Autodesk Inventor part; units mm, degrees
ref_plane "YZ Plane" through (0, 0, 0) normal (1, 0, 0) x (0, 1, 0)
ref_plane "XZ Plane" through (0, 0, 0) normal (0, 1, 0) x (-1, 0, 0)
ref_plane "XY Plane" through (0, 0, 0) normal (0, 0, 1) x (1, 0, 0)
ref_plane "РабПлоскость1" through (0, 0, 0) normal (0, 0, 1) x (1, 0, 0)
sketch "Эскиз1" plane through (0, 0, 0) normal (0, 0, 1) x (1, 0, 0)
  circle A0 centre (0, 0) radius 10
  dimension "d0" = 20
extrude "Выдавливание1" add sketch "Эскиз1" against normal blind 90
sketch "Эскиз2" plane through (0, 0, 0) normal (0, 0, 1) x (1, 0, 0)
  circle A0 centre (0, 0) radius 15
  dimension "d3" = 30
extrude "Выдавливание2" add sketch "Эскиз2" along normal blind 30
chamfer "Фаска1" distance 2 angle 45 2 edges at (-15, 0, 30) (-10, 0, -90)
ref_plane "РабПлоскость2" through (-11.5, 3, -60) normal (1, 0, 0) x (0, 1, 0)
sketch "Эскиз3" plane through (-11.5, 3, -60) normal (1, 0, 0) x (0, 1, 0)
  line L0 (-18, 60) -> (12, 60)
  line L1 (12, 88) -> (-18, 88)
  line L2 (-13, 60) -> (7, 60)
  line L3 (-13, -28) -> (7, -28)
  line L4 (-3, 10) -> (-3, 10)
  line L5 (0, 13) -> (0, 47)
  line L6 (-3, 50) -> (-3, 50)
  line L7 (-6, 47) -> (-6, 13)
  line L8 (-6, 10) -> (0, 50) construction
  line L9 (0, 10) -> (-6, 50) construction
  arc A0 (0, 47) -> (-3, 50) centre (-3, 47) ccw
  arc A1 (-3, 50) -> (-6, 47) centre (-3, 47) ccw
  arc A2 (-3, 10) -> (0, 13) centre (-3, 13) ccw
  arc A3 (-6, 13) -> (-3, 10) centre (-3, 13) ccw
  point P0 (-3, 60)
  point P1 (-3, 30)
  dimension "d9" = 30
  dimension "d10" = 6
  dimension "d11" = 40
  dimension "d12" = 3
extrude "Выдавливание3" cut sketch "Эскиз3" along normal blind 6
properties part number "Ось"
Check sheet for the modelled part. Datum: model origin and axes. Units: mm. A direction names the side the tool comes from. Round coordinates to 2 decimals unless told otherwise and drop trailing zeros. Order: outer loops, then holes, each group sorted by start corner. A loop starts at its lowest first (then second) coordinate and runs counter-clockwise, first axis right, second up.
1) Section check C-C (z = -34.5). Record the boundary of the cut face in (x, y).
2) Go/stop test with flat-tipped pins: pin 1 Ø5 at (x, z) = (10.5, -7) entering from -Y; pin 2 Ø8 at (x, z) = (4.5, -46.5) entering from -Y; pin 3 Ø4 at (y, z) = (1.5, -67) entering from -X. Record where each tip stops, or that it passes through.
3) Section check D-D (z = -67.5). Record the boundary of the cut face in (x, y).
4) Scan lines: line 1 (X direction, y = -0.75, z = 21); line 2 (Z direction, x = 7.25, y = 9); line 3 (X direction, y = -0.5, z = -4.5). Record each from-to range of solid material in increasing order.
5) Section check B-B (y = 0). Record the boundary of the cut face in (x, z).
6) Tool access check on faces 1 (the conical face through (-2.845, 12.813, 29.875)), 2 (the cylindrical face through (9.54, 3, -43.38)), 3 (the cylindrical face through (-8, 0, -50)). Record the directions out of +Z, -Z, +X, -X, +Y, -Y that give a thin tool (end or side, any length) a straight path to the whole face; none if there is none.
7) Mould release check, pull along Z, two halves, no side actions. Record for faces 4 (the flat face through (0, 0, 30)), 5 (the flat face through (3, -10, 0)), 6 (the cylindrical face through (-14.985, -0.66, 13.804)), 7 (the cylindrical face through (-8, 0, -10)): +Z half, -Z half, draft (parallel to the pull), parting line (faces both ways), or undercut.
8) Section check A-A (x = 0). Record the boundary of the cut face in (y, z), and give its area (3 significant figures).
Result:
1. outline: (-9.54, -3) arc R10 ccw (long way) to (-9.54, 3) - (-5.5, 3) - (-5.5, -3) - close
2. pin 1: stops at y = -6
2. pin 2: stops at y = -9.99
2. pin 3: stops at x = -10
3. outline: circle Ø20 at (0, 0)
4. line 1: x = -14.98 to 14.98
4. line 2: z = 0 to 30
4. line 3: x = -9.99 to 9.99
5. outline: (-15, 0) - (-10, 0) - (-10, -10) - (-5.5, -10) - (-5.5, -50) - (-10, -50) - (-10, -88) - (-8, -90) - (8, -90) - (10, -88) - (10, 0) - (15, 0) - (15, 28) - (13, 30) - (-13, 30) - (-15, 28) - close
6. face 1: +Z
6. face 2: -Z
6. face 3: -X
7. face 4: +Z half
7. face 5: -Z half
7. face 6: draft
7. face 7: undercut
8. outline: (-15, 0) - (-10, 0) - (-10, -88) - (-8, -90) - (8, -90) - (10, -88) - (10, 0) - (15, 0) - (15, 28) - (13, 30) - (-13, 30) - (-15, 28) - close
8. area: 2,690 mm2
